Study the drawing (mm; zero at the part's minimum x, y, z) and answer. Give positions to 0.01 mm unless a question says otherwise; leave off trailing zeros. Order: outer loops, then holes, each group sorted by start corner. A loop starts at its lowest first (then second) coordinate and runs counter-clockwise, first axis right, second up.
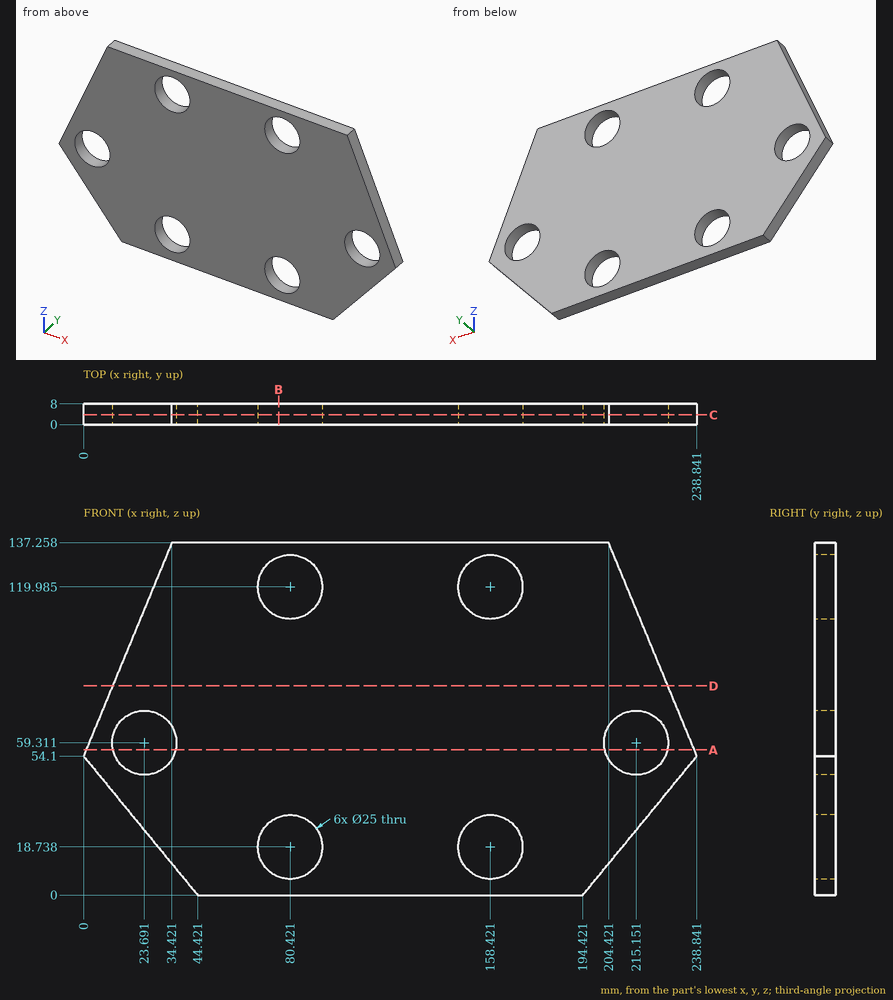
1) Find section D-D (z = 81.5). Write down the section's boundary in (x, y).
Geometry says:
outline: (11.34, 0) - (227.5, 0) - (227.5, 8) - (11.34, 8) - close
2) Find section C-C (y = 3.75). Count the separate pieces of the cut face and the enclosed holes in it, then the cut area to 3 significant figures.
Geometry says:
separate pieces: 1
enclosed holes: 6
area: 24,600 mm2
3) Find section B-B (x = 76). Write down the section's boundary in (y, z) (1 decimal).
Geometry says:
outline: (0, 0) - (8, 0) - (8, 7) - (0, 7) - close; (0, 30.4) - (8, 30.4) - (8, 108.3) - (0, 108.3) - close; (0, 131.7) - (8, 131.7) - (8, 137.3) - (0, 137.3) - close
4) Straight lines are drawn through the part: probe 1 along Z at (x, y) = (161, 5) (1 decimal); probe 2 along X at (y, z) = (4, 116); probe 3 along X at (y, z) = (0.5, 125) (1 decimal). For each, find the intervals that lie inside material, in ascending order.
Geometry says:
probe 1: z = 0 to 6.5, 31 to 107.8, 132.2 to 137.3
probe 2: x = 25.62 to 68.57, 92.27 to 146.57, 170.27 to 213.22
probe 3: x = 29.3 to 69, 91.9 to 147, 169.9 to 209.5
5) Given P1, Ø4, axis at y = 3, z = 86, coming from the -X side; P2, Ø20, axis at x = 158.42, z = 119.99, coming from the +Y side; P3, Ø3, axis at y = 2.5, z = 34.5, coming from the -X side; P4, Ø4, axis at x = 40.5, y = 2.5, coming from the -Z side, each flat-ended and moving along its own axis, determine where each tip first touches the part or whether it passes through.
Geometry says:
P1: stops at x = 12.38
P2: passes through
P3: stops at x = 14.86
P4: stops at z = 2.34
6) Find section A-A (z = 56.5). Write down the section's boundary in (x, y).
Geometry says:
outline: (0.99, 0) - (11.51, 0) - (11.51, 8) - (0.99, 8) - close; (35.87, 0) - (202.97, 0) - (202.97, 8) - (35.87, 8) - close; (227.33, 0) - (237.85, 0) - (237.85, 8) - (227.33, 8) - close
